Could you check a few things on this model? Use its own coordinates, in mm. Round coordinates to 2 decimals unless told otherwise and drop trailing zeros. Loops run counter-clockwise (first coordinate to the right, second up) from the corner with the lowest first, then second, coordinate; pieces in that order, holes last. Notation, with made-up numbers: (3.25, -11.5) -> (25.25, -11.5) arc R23 cw to (25.25, -3.5) -> close; hole circle Ø9 at (71, -14). An arc over 180 degrees is marked (long way). Use CSV: the item, a comma, the result in double quotes. Start each with the question number.
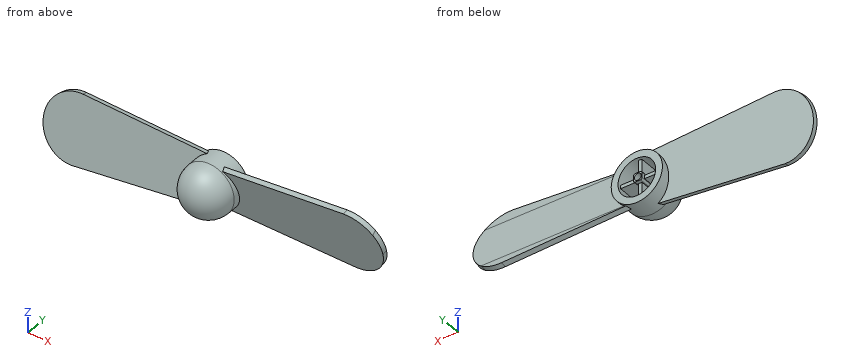
```python
from build123d import *

# Parameters (mm, degrees)
SKETCH_1_R               = 7.5
EXTRUDE_1_DEPTH          = 6
EXTRUDE_2_DEPTH          = 50
EXTRUDE_3_DEPTH          = 1.5
CUT_EXTRUDE_START        = -1.5
CUT_EXTRUDE_2_DEPTH      = 1.475557967
PATTERN_CIRCULAR_1_COUNT = 2
REVOLVE_1_ANGLE          = 180
EXTRUDE_5_REACH          = 54.77
SKETCH_8_W               = 2.5
SKETCH_8_H               = 2.5
EXTRUDE_6_REACH          = 55.77
EXTRUDE_START            = -1
SKETCH_14_W              = 6.185620564
SKETCH_14_H              = 1
EXTRUDE_7_REACH          = 54.523
SKETCH_15_W              = 1
SKETCH_15_H              = 5.873847005
FILLET_1_R               = 0.5
SKETCH_16_R              = 1
CUT_EXTRUDE_5_DEPTH      = 7


# Read off the part's stored shape, not the designer's step: 切除-拉伸2, 抽壳9
with BuildPart() as part:
    # 草图1 → 凸台-拉伸1 (new body)
    with BuildSketch(Plane(origin=(0, 0, 0), x_dir=(1, 0, 0), z_dir=(0, 1, 0))):
        with Locations(Location((0.301002806, -0.075250701, 0), (0, 0, 270))):
            Circle(SKETCH_1_R)
    extrude(amount=EXTRUDE_1_DEPTH)

    # 草图2 → 凸台-拉伸2 (add)
    with BuildSketch(Plane(origin=(0, 0, 0), x_dir=(0, 0, -1), z_dir=(1, 0, 0))):
        Polygon((-6.841656071, 1.896781733), (-6.217832024, 0.532654335), (6.742880936, 3.816427212), (6.11905689, 5.18055461), align=None)
    extrude(amount=EXTRUDE_2_DEPTH)

    # 草图3 → 凸台-拉伸3 (add)
    with BuildSketch(Plane(origin=(0, 3.411230811, 0.864281714), x_dir=(1, 0, 0), z_dir=(0, 0.9693704528417939, 0.24560318637447578))):
        with BuildLine():
            Line((3.425595735, 7.47367623), (3.536085243, -6.166243606))
            Line((3.536085243, -6.166243606), (40.104138222, -9.535908549))
            ThreePointArc((40.104138222, -9.535908549), (50, -0.119655983), (40.104138222, 9.296596584))
            Line((40.104138222, 9.296596584), (3.425595735, 7.47367623))
        make_face()
    extrude_3 = extrude(amount=-EXTRUDE_3_DEPTH)

    # 切除-拉伸2 outline → 切除-拉伸2 (cut)
    with BuildSketch(Plane(origin=(0, 1.957175132, 0.495876935), x_dir=(1, 0, 0), z_dir=(0, -0.9693704528417938, -0.24560318637447576)).offset(CUT_EXTRUDE_START)):
        with BuildLine():
            Line((59.770521771, 9.535908549), (41.04011208, 9.535908549))
            ThreePointArc((41.04011208, 9.535908549), (47.402093905, 6.618605973), (50, 0.119655983))
            ThreePointArc((50, 0.119655983), (47.402093905, -6.379294008), (41.040112081, -9.296596584))
            Line((41.040112081, -9.296596584), (60.303287448, -9.296596584))
            Line((60.303287448, -9.296596584), (59.770521771, 9.535908549))
        make_face()
    extrude(amount=CUT_EXTRUDE_2_DEPTH, mode=Mode.SUBTRACT)

    # 阵列(圆周)1: 凸台-拉伸3 ×2 about axis
    pattern_circular_1_axis = Axis((0.301002806, 0, 0.075250701), (0, 1, 0))
    for i in range(1, PATTERN_CIRCULAR_1_COUNT):
        add(extrude_3.rotate(pattern_circular_1_axis, i * 360 / PATTERN_CIRCULAR_1_COUNT))

    # 草图6 → 旋转1 (revolve)
    with BuildSketch(Plane(origin=(0, 0, 0), x_dir=(1, 0, 0), z_dir=(0, 1, 0))):
        with BuildLine():
            Line((7.577071557, -1.894267889), (-6.975065945, 1.743766486))
            ThreePointArc((-6.975065945, 1.743766486), (2.120019994, 7.20081805), (7.577071557, -1.894267889))
        make_face()
    revolve(axis=Axis((7.577071557, 0, 1.894267889), (-0.9701425001453376, 0, -0.2425356250363098)), revolution_arc=REVOLVE_1_ANGLE)

    # 抽壳9 outline → 抽壳9 (revolve, cut)
    with BuildSketch(Plane(origin=(0.301002806, 0, 0.075250701), x_dir=(1, 0, 0), z_dir=(0, 0, 1))):
        with BuildLine():
            Line((5.5, 6e-09), (5.5, 6))
            Line((5.5, 6), (0, 6))
            Line((0, 6), (0, -5.5))
            ThreePointArc((0, -5.5), (3.889087299, -3.889087294), (5.5, 6e-09))
        make_face()
    revolve(axis=Axis((0.301002806, 0, 0.075250701), (0, 1, 0)), mode=Mode.SUBTRACT)

    # 草图8 → 凸台-拉伸5 (add, up to next)
    with BuildSketch(Plane(origin=(0, 6, 0), x_dir=(1, 0, 0), z_dir=(0, 1, 0)), mode=Mode.PRIVATE) as extrude_5_sk1:
        Rectangle(SKETCH_8_W, SKETCH_8_H)
    extrude_5_tool1 = extrude(extrude_5_sk1.sketch, amount=-EXTRUDE_5_REACH, mode=Mode.PRIVATE) - part.part
    add(extrude_5_tool1.solids().sort_by_distance((0, 6, 0))[0])

    # 草图14 → 凸台-拉伸6 (add, up to next)
    with BuildSketch(Plane(origin=(0, 6, 0), x_dir=(1, 0, 0), z_dir=(0, 1, 0)).offset(EXTRUDE_START), mode=Mode.PRIVATE) as extrude_6_sk1:
        with Locations((3.092810282, 0)):
            Rectangle(SKETCH_14_W, SKETCH_14_H)
    extrude_6_tool1 = extrude(extrude_6_sk1.sketch, amount=-EXTRUDE_6_REACH, mode=Mode.PRIVATE) - part.part
    extrude_6 = extrude_6_tool1.solids().sort_by_distance((3.09281, 5, 0))[0]
    add(extrude_6)

    # 镜向1: 凸台-拉伸6 across plane
    add(extrude_6.mirror(Plane(origin=(0, 0, 0), x_dir=(0, 0, 1), z_dir=(1, 0, 0))))

    # 草图15 → 凸台-拉伸7 (add, up to next)
    with BuildSketch(Plane(origin=(0, 5, 0), x_dir=(1, 0, 0), z_dir=(0, 1, 0)), mode=Mode.PRIVATE) as extrude_7_sk1:
        with Locations((0, 2.936923503)):
            Rectangle(SKETCH_15_W, SKETCH_15_H)
    extrude_7_tool1 = extrude(extrude_7_sk1.sketch, amount=-EXTRUDE_7_REACH, mode=Mode.PRIVATE) - part.part
    extrude_7 = extrude_7_tool1.solids().sort_by_distance((0, 5, -2.936924))[0]
    add(extrude_7)

    # 镜向2: 凸台-拉伸7 mirrored; each copy of 凸台-拉伸7 runs up to whatever stops it at its own place
    mirror_2_before = part.part  # the part as the pattern finds it: every copy runs up to it
    mirror_2_extrude_7_long = extrude(extrude_7_sk1.sketch, amount=-EXTRUDE_7_REACH, mode=Mode.PRIVATE)
    mirror_2_extrude_7_tool1 = mirror_2_extrude_7_long.mirror(Plane.XY) - mirror_2_before
    add(mirror_2_extrude_7_tool1.solids().sort_by_distance((0, 5, 2.936924))[0])

    # 圆角1
    fillet_1_edges = [part.edges().sort_by_distance(p)[0] for p in [
        (-1.25, 0.427824152, 1.25),
        (1.25, 0.355696292, 1.25),
        (1.25, 0.373542552, -1.25),
        (-1.25, 0.446174395, -1.25),
    ]]
    fillet(fillet_1_edges, radius=FILLET_1_R)

    # 草图16 → 切除-拉伸5 (cut)
    with BuildSketch(Plane(origin=(0, 6, 0), x_dir=(1, 0, 0), z_dir=(0, 1, 0))):
        with Locations(Location((0, 0, 0), (0, 0, 270))):
            Circle(SKETCH_16_R)
    extrude(amount=-CUT_EXTRUDE_5_DEPTH, mode=Mode.SUBTRACT)


solid = part.part
```
1. Suppose I cut it at A-A (x = 33). List the corners of the cut face in (y, z) for me.
2. If I drill on L1, parallel to X at y = 1.25, z = -3.5; L2, parallel to X at y = 4.25, z = 0; L3, parallel to X at y = -2.5, z = -4, over which ranges is the centre line in solid material (lowest first)?
3. Will these pins go through, and if not, where does the flat tip stop? pin 1 (4 mm diameter, centred on x = -36.5, y = 4, fed in from +Z); pin 2 (0.5 mm diameter, centred on x = 0, y = -2, fed in from +Z); pin 3 (1.1 mm diameter, centred on x = 0, z = 4, fed in from +Y).
Geometry check:
1,outline,"(-0.22, 9.11) -> (4.15, -8.17) -> (5.61, -7.81) -> (1.23, 9.47) -> close"
2,L1,"x = -48.87 to -3.88, -0.5 to 0.5, 4.48 to 6.89"
2,L2,"x = -7.2 to -1, 1 to 7.8"
2,L3,"x = -5.48 to -2.42, -0.5 to 0.5, 3.02 to 6.08"
3,pin 1,"stops at z = 8.62"
3,pin 2,"stops at z = 7.36"
3,pin 3,"stops at y = 5"
